```python
from build123d import *

# Parameters (mm, degrees)
F0_R        = 4.2
F1_DEPTH    = 3
F3_DEPTH    = 3
F4_R        = 5
F5_T1_DEPTH = 3


# Not quite as in the source:
# - a fillet or chamfer that OpenCascade refuses, or shapes differently, is made with other operations: its cross-section is extruded or revolved along the edge and cut away or added


with BuildPart() as f1:
    # F0 (on Top) → F1 (new body)
    with BuildSketch(Plane.XY):
        with BuildLine():
            ThreePointArc((6.5452272688, 3), (7.0344024741, 1.5353116402), (7.2, 0))
            Line((7.2, 0), (33, 0))
            Line((33, 0), (36, 0))
            Line((36, 0), (61.8, 0))
            ThreePointArc((61.8, 0), (61.9655975259, 1.5353116402), (62.4547727312, 3))
            Line((62.4547727312, 3), (39.1503768868, 3))
            ThreePointArc((39.1503768868, 3), (69, 30), (98.8496231132, 3))
            Line((98.8496231132, 3), (75.5452272688, 3))
            ThreePointArc((75.5452272688, 3), (76.0344024741, 1.5353116402), (76.2, 0))
            Line((76.2, 0), (102, 0))
            ThreePointArc((102, 0), (79.5543660777, 31.2666812549), (42.7511905032, 20))
            Line((42.7511905032, 20), (26.2488094968, 20))
            ThreePointArc((26.2488094968, 20), (-10.5543660777, 31.2666812549), (-33, 0))
            Line((-33, 0), (-7.2, 0))
            ThreePointArc((-7.2, 0), (-7.0344024741, 1.5353116402), (-6.5452272688, 3))
            Line((-6.5452272688, 3), (-29.8496231132, 3))
            ThreePointArc((-29.8496231132, 3), (0, 30), (29.8496231132, 3))
            Line((29.8496231132, 3), (6.5452272688, 3))
        make_face()
        with BuildLine():
            Line((36.1366465497, 3), (32.8633534503, 3))
            ThreePointArc((32.8633534503, 3), (31.364916731, 10.2587522855), (28.2842712475, 17))
            Line((28.2842712475, 17), (40.7157287525, 17))
            ThreePointArc((40.7157287525, 17), (37.635083269, 10.2587522855), (36.1366465497, 3))
        make_face(mode=Mode.SUBTRACT)
        with BuildLine():
            ThreePointArc((-7.2, 0), (0, -7.2), (7.2, 0))
            ThreePointArc((7.2, 0), (7.0344024741, 1.5353116402), (6.5452272688, 3))
            ThreePointArc((6.5452272688, 3), (0, 7.2), (-6.5452272688, 3))
            ThreePointArc((-6.5452272688, 3), (-7.0344024741, 1.5353116402), (-7.2, 0))
        make_face()
        Circle(F0_R, mode=Mode.SUBTRACT)
        with BuildLine():
            ThreePointArc((62.4547727312, 3), (61.9655975259, 1.5353116402), (61.8, 0))
            ThreePointArc((61.8, 0), (69, -7.2), (76.2, 0))
            ThreePointArc((76.2, 0), (76.0344024741, 1.5353116402), (75.5452272688, 3))
            ThreePointArc((75.5452272688, 3), (69, 7.2), (62.4547727312, 3))
        make_face()
        with Locations((69, 0)):
            Circle(F0_R, mode=Mode.SUBTRACT)
    extrude(amount=F1_DEPTH)

    # F2 (on face) → F3 (join, through all)
    with BuildSketch(Plane.XY.offset(3)):
        with BuildLine():
            Line((1.5, 7.0420167566), (1.5, 29.9624765332))
            ThreePointArc((1.5, 29.9624765332), (0.7502346317, 29.9906176662), (0, 30))
            Line((0, 30), (0, 7.2))
            ThreePointArc((0, 7.2), (0.7541483119, 7.1603952631), (1.5, 7.0420167566))
        make_face()
        with BuildLine():
            Line((0, 7.2), (0, 30))
            ThreePointArc((0, 30), (-0.7502346317, 29.9906176662), (-1.5, 29.9624765332))
            Line((-1.5, 29.9624765332), (-1.5, 7.0420167566))
            ThreePointArc((-1.5, 7.0420167566), (-0.7541483119, 7.1603952631), (0, 7.2))
        make_face()
        with BuildLine():
            Line((69, 7.2), (69, 30))
            ThreePointArc((69, 30), (68.2497653683, 29.9906176662), (67.5, 29.9624765332))
            Line((67.5, 29.9624765332), (67.5, 7.0420167566))
            ThreePointArc((67.5, 7.0420167566), (68.2458516881, 7.1603952631), (69, 7.2))
        make_face()
        with BuildLine():
            Line((70.5, 7.0420167566), (70.5, 29.9624765332))
            ThreePointArc((70.5, 29.9624765332), (69.7502346317, 29.9906176662), (69, 30))
            Line((69, 30), (69, 7.2))
            ThreePointArc((69, 7.2), (69.7541483119, 7.1603952631), (70.5, 7.0420167566))
        make_face()
    extrude(amount=-F3_DEPTH)

    # F4
    f4_edges = [f1.edges().sort_by_distance(p)[0] for p in [
        (-29.849623, 3, 1.5),
        (29.849623, 3, 1.5),
        (98.849623, 3, 1.5),
        (39.150377, 3, 1.5),
        (-7.2, 0, 1.5),
        (7.2, 0, 1.5),
        (61.8, 0, 1.5),
        (76.2, 0, 1.5),
        (75.545227, 3, 1.5),
        (62.454773, 3, 1.5),
        (-6.545227, 3, 1.5),
        (6.545227, 3, 1.5),
        (26.248809, 20, 1.5),
        (42.751191, 20, 1.5),
        (102, 0, 1.5),
        (-33, 0, 1.5),
        (-1.5, 7.042017, 1.5),
        (1.5, 7.042017, 1.5),
        (1.5, 29.962477, 1.5),
        (-1.5, 29.962477, 1.5),
        (70.5, 29.962477, 1.5),
        (67.5, 29.962477, 1.5),
    ]]
    fillet(f4_edges, radius=F4_R)

    # F5: fillet of radius 2 on 4 edges, made by hand

    # F5_s2 → F5_t1 (join)
    with BuildSketch(Plane.XY):
        with BuildLine():
            ThreePointArc((31.6227766017, 17), (29.9324680922, 16.0690449676), (29.8157607959, 14.1428571429))
            ThreePointArc((29.8157607959, 14.1428571429), (29.0851207181, 15.5902454379), (28.2842712475, 17))
            Line((28.2842712475, 17), (31.6227766017, 17))
        make_face()
        with BuildLine():
            ThreePointArc((37.3772233983, 17), (39.0675319078, 16.0690449676), (39.1842392041, 14.1428571429))
            ThreePointArc((39.1842392041, 14.1428571429), (39.9148792819, 15.5902454379), (40.7157287525, 17))
            Line((40.7157287525, 17), (37.3772233983, 17))
        make_face()
        with BuildLine():
            ThreePointArc((34.6410161514, 3), (33.33170881, 3.488142108), (32.6615295142, 4.7142857143))
            ThreePointArc((32.6615295142, 4.7142857143), (32.7736520051, 3.8584626791), (32.8633534503, 3))
            Line((32.8633534503, 3), (34.6410161514, 3))
        make_face()
        with BuildLine():
            ThreePointArc((36.3384704858, 4.7142857143), (35.66829119, 3.488142108), (34.3589838486, 3))
            Line((34.3589838486, 3), (36.1366465497, 3))
            ThreePointArc((36.1366465497, 3), (36.2263479949, 3.8584626791), (36.3384704858, 4.7142857143))
        make_face()
    extrude(amount=F5_T1_DEPTH)


solid = f1.part
```
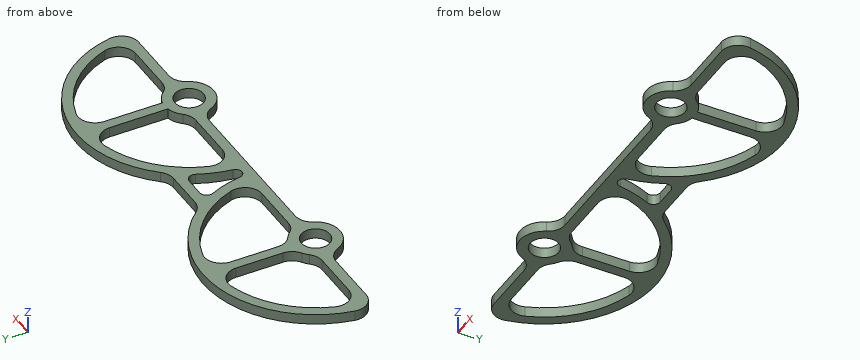
Design review of the part built by this model. Coordinates are the model's own, in mm. Coordinates: 2 decimals unless noted, no trailing zeros. Write each loop counter-clockwise with the first axis right and the second up, starting at its lowest first coordinate (ties: lowest second). Pieces come first, ordered by that corner, then holes.
1) To check wall thickness, follow L1, parallel to X at y = 21, z = 2.45; L2, parallel to Y at x = 69, z = 2.1; L3, parallel to X at y = 13, z = 0.5. State the ranges of each line that lie inside material, in increasing order.
2) Insertion check: pin 1 (0.9 mm diameter, centred on x = 30.5, z = 1, fed in from -Y); pin 2 (1.5 mm diameter, centred on x = 87, z = 1.5, fed in from +Y); pin 3 (1.5 mm diameter, centred on y = 11.5, z = 1, fed in from -X); pin 4 (10 mm diameter, centred on x = 42, y = 15.5, fed in from -Z). Each pin has a flat end and moves straight along its axis. Give the tip position at first contact, or say it passes through.
3) Add section A-A (x = 69). Write out the cut boundary in (y, z), plus the area to 3 significant figures.
4) Add section C-C (z = 1.5). State how many separate pieces and enclosed holes the cut face has, plus the area to 3 significant figures.
5) Add section D-D (x = -14.5). Write out the cut boundary in (y, z), plus the area to 3 significant figures.
6) Add section B-B (y = 23). Write out the cut boundary in (x, z).
Check result:
1. L1: x = -25.46 to -21.42, -1.5 to 1.5, 21.42 to 25.62, 43.38 to 47.58, 67.5 to 70.5, 90.42 to 94.46
1. L2: y = -7.2 to -4.2, 4.2 to 33
1. L3: x = -30.33 to -27.04, -1.5 to 1.5, 27.04 to 30.33, 38.67 to 41.96, 67.5 to 70.5, 96.04 to 99.33
2. pin 1: stops at y = 0
2. pin 2: stops at y = 28.13
2. pin 3: stops at x = -31.2
2. pin 4: stops at z = 0
3. outline: (-7.2, 0) - (-4.2, 0) - (-4.2, 3) - (-7.2, 3) - close; (4.2, 0) - (33, 0) - (33, 3) - (4.2, 3) - close
3. area: 95.4 mm2
4. separate pieces: 1
4. enclosed holes: 7
4. area: 1,350 mm2
5. outline: (0, 0) - (3, 0) - (3, 3) - (0, 3) - close; (26.26, 0) - (29.64, 0) - (29.64, 3) - (26.26, 3) - close
5. area: 19.1 mm2
6. outline: (-23.66, 0) - (-19.26, 0) - (-19.26, 3) - (-23.66, 3) - close; (-1.5, 0) - (1.5, 0) - (1.5, 3) - (-1.5, 3) - close; (19.26, 0) - (23.66, 0) - (23.66, 3) - (19.26, 3) - close; (45.34, 0) - (49.74, 0) - (49.74, 3) - (45.34, 3) - close; (67.5, 0) - (70.5, 0) - (70.5, 3) - (67.5, 3) - close; (88.26, 0) - (92.66, 0) - (92.66, 3) - (88.26, 3) - close
